```python
from build123d import *

# Parameters (mm, degrees)
SCHIZZO1_W                   = 470
SCHIZZO1_H                   = 100
SCHIZZO1_R                   = 35
ESTRUSIONE_ESTRUSIONE1_DEPTH = 5
FORO_PER_VITE_M8_1_D         = 8.5
RIPETIZIONECIRCOLARE1_COUNT  = 8
SCHIZZO6_R                   = 28
TAGLIO_ESTRUSIONE1_DEPTH     = 3
SMUSSO1_SIZE                 = 0.5
SCHIZZO7_R                   = 2.75
TAGLIO_ESTRUSIONE2_DEPTH     = 424.083916026
RIPETIZIONECIRCOLARE2_COUNT  = 6
RACCORDO1_R                  = 20
RACCORDO2_R                  = 50
TAGLIO_ESTRUSIONE3_START     = -10
TAGLIO_ESTRUSIONE3_DEPTH     = 4
SCHIZZO10_R                  = 2.1
TAGLIO_ESTRUSIONE4_DEPTH     = 424.083916026
SCHIZZO11_R                  = 3.4
TAGLIO_ESTRUSIONE5_DEPTH     = 10
SCHIZZO12_R                  = 2.1
TAGLIO_ESTRUSIONE6_DEPTH     = 424.083916026
TAGLIO_ESTRUSIONE7_DEPTH     = 424.008274151


with BuildPart() as part:
    # Schizzo1 → Estrusione-Estrusione1 (new, symmetric)
    with BuildSketch(Plane(origin=(0, 0, 0), x_dir=(1, 0, 0), z_dir=(0, 1, 0))):
        with Locations((-185, 0)):
            Rectangle(SCHIZZO1_W, SCHIZZO1_H)
        with Locations(Location((-370, 0, 0), (0, 0, 270))):
            Circle(SCHIZZO1_R, mode=Mode.SUBTRACT)
    extrude(amount=ESTRUSIONE_ESTRUSIONE1_DEPTH, both=True)

    # Foro per Vite M8-1 (through all)
    with Locations(Plane(origin=(0, 5, 0), x_dir=(1, 0, 0), z_dir=(0, 1, 0))):
        with Locations((21, 0)):
            foro_per_vite_m8_1 = Hole(FORO_PER_VITE_M8_1_D / 2)

    # RipetizioneCircolare1: Foro per Vite M8-1 ×8 about axis
    ripetizionecircolare1_axis = Axis((0, 0, 0), (0, 1, 0))
    for i in range(1, RIPETIZIONECIRCOLARE1_COUNT):
        add(foro_per_vite_m8_1.rotate(ripetizionecircolare1_axis, i * 360 / RIPETIZIONECIRCOLARE1_COUNT), mode=Mode.SUBTRACT)

    # Schizzo6 → Taglio-Estrusione1 (cut)
    with BuildSketch(Plane.XZ.offset(5)):
        with Locations(Location((0, 0, 0), (0, 0, 270))):
            Circle(SCHIZZO6_R)
    extrude(amount=-TAGLIO_ESTRUSIONE1_DEPTH, mode=Mode.SUBTRACT)

    # Smusso1
    smusso1_edges = [part.edges().sort_by_distance(p)[0] for p in [
        (0, -5, 28),
    ]]
    chamfer(smusso1_edges, length=SMUSSO1_SIZE)

    # Schizzo7 → Taglio-Estrusione2 (cut, through all)
    with BuildSketch(Plane(origin=(0, 5, 0), x_dir=(1, 0, 0), z_dir=(0, 1, 0))):
        with Locations(Location((-370, 41, 0), (0, 0, 270))):
            Circle(SCHIZZO7_R)
    taglio_estrusione2 = extrude(amount=-TAGLIO_ESTRUSIONE2_DEPTH, mode=Mode.SUBTRACT)

    # RipetizioneCircolare2: Taglio-Estrusione2 ×6 about axis
    ripetizionecircolare2_axis = Axis((-370, 0, 0), (0, 1, 0))
    for i in range(1, RIPETIZIONECIRCOLARE2_COUNT):
        add(taglio_estrusione2.rotate(ripetizionecircolare2_axis, i * 360 / RIPETIZIONECIRCOLARE2_COUNT), mode=Mode.SUBTRACT)

    # Raccordo1
    raccordo1_edges = [part.edges().sort_by_distance(p)[0] for p in [
        (50, 0, -50),
        (50, 0, 50),
    ]]
    fillet(raccordo1_edges, radius=RACCORDO1_R)

    # Raccordo2
    raccordo2_edges = [part.edges().sort_by_distance(p)[0] for p in [
        (-420, 0, -50),
        (-420, 0, 50),
    ]]
    fillet(raccordo2_edges, radius=RACCORDO2_R - 0.0001)  # a hair under: the kernel refuses the full size

    # Schizzo9 → Taglio-Estrusione3 (cut)
    with BuildSketch(Plane(origin=(0, 5, 0), x_dir=(1, 0, 0), z_dir=(0, 1, 0)).offset(TAGLIO_ESTRUSIONE3_START)):
        with BuildLine():
            Line((-32, 46.55), (-20, 46.55))
            ThreePointArc((-20, 46.55), (-15.95, 42.5), (-20, 38.45))
            Line((-20, 38.45), (-32, 38.45))
            ThreePointArc((-32, 38.45), (-36.05, 42.5), (-32, 46.55))
        make_face()
        with BuildLine():
            Line((20, 46.55), (32, 46.55))
            ThreePointArc((32, 46.55), (36.05, 42.5), (32, 38.45))
            Line((32, 38.45), (20, 38.45))
            ThreePointArc((20, 38.45), (15.95, 42.5), (20, 46.55))
        make_face()
        with BuildLine():
            Line((-32, -38.45), (-20, -38.45))
            ThreePointArc((-20, -38.45), (-15.95, -42.5), (-20, -46.55))
            Line((-20, -46.55), (-32, -46.55))
            ThreePointArc((-32, -46.55), (-36.05, -42.5), (-32, -38.45))
        make_face()
        with BuildLine():
            Line((20, -38.45), (32, -38.45))
            ThreePointArc((32, -38.45), (36.05, -42.5), (32, -46.55))
            Line((32, -46.55), (20, -46.55))
            ThreePointArc((20, -46.55), (15.95, -42.5), (20, -38.45))
        make_face()
    extrude(amount=TAGLIO_ESTRUSIONE3_DEPTH, mode=Mode.SUBTRACT)

    # Schizzo10 → Taglio-Estrusione4 (cut, through all)
    with BuildSketch(Plane(origin=(0, 5, 0), x_dir=(1, 0, 0), z_dir=(0, 1, 0))):
        with Locations(Location((-150, 0, 0), (0, 0, 270))):
            Circle(SCHIZZO10_R)
    extrude(amount=-TAGLIO_ESTRUSIONE4_DEPTH, mode=Mode.SUBTRACT)

    # Schizzo11 → Taglio-Estrusione5 (cut)
    with BuildSketch(Plane(origin=(0, 5, 0), x_dir=(1, 0, 0), z_dir=(0, 1, 0))):
        with Locations(Location((-280, 43.588989435, 0), (0, 0, 270))):
            Circle(SCHIZZO11_R)
    extrude(amount=-TAGLIO_ESTRUSIONE5_DEPTH, mode=Mode.SUBTRACT)

    # Schizzo12 → Taglio-Estrusione6 (cut, through all)
    with BuildSketch(Plane(origin=(0, 5, 0), x_dir=(1, 0, 0), z_dir=(0, 1, 0))):
        with Locations(Location((-50, -42.5, 0), (0, 0, 270))):
            Circle(SCHIZZO12_R)
        with Locations(Location((-300, -42.5, 0), (0, 0, 270))):
            Circle(SCHIZZO12_R)
        with Locations(Location((-175, -42.5, 0), (0, 0, 270))):
            Circle(SCHIZZO12_R)
    extrude(amount=-TAGLIO_ESTRUSIONE6_DEPTH, mode=Mode.SUBTRACT)

    # Schizzo13 → Taglio-Estrusione7 (cut, through all)
    with BuildSketch(Plane(origin=(0, -1, 0), x_dir=(-1, 0, 0), z_dir=(0, -1, 0))):
        with BuildLine():
            Line((32, -45.25), (20, -45.25))
            ThreePointArc((20, -45.25), (17.25, -42.5), (20, -39.75))
            Line((20, -39.75), (32, -39.75))
            ThreePointArc((32, -39.75), (34.75, -42.5), (32, -45.25))
        make_face()
        with BuildLine():
            Line((-20, -45.25), (-32, -45.25))
            ThreePointArc((-32, -45.25), (-34.75, -42.5), (-32, -39.75))
            Line((-32, -39.75), (-20, -39.75))
            ThreePointArc((-20, -39.75), (-17.25, -42.5), (-20, -45.25))
        make_face()
        with BuildLine():
            Line((-32, 45.25), (-20, 45.25))
            ThreePointArc((-20, 45.25), (-17.25, 42.5), (-20, 39.75))
            Line((-20, 39.75), (-32, 39.75))
            ThreePointArc((-32, 39.75), (-34.75, 42.5), (-32, 45.25))
        make_face()
        with BuildLine():
            Line((20, 45.25), (32, 45.25))
            ThreePointArc((32, 45.25), (34.75, 42.5), (32, 39.75))
            Line((32, 39.75), (20, 39.75))
            ThreePointArc((20, 39.75), (17.25, 42.5), (20, 45.25))
        make_face()
    extrude(amount=-TAGLIO_ESTRUSIONE7_DEPTH, mode=Mode.SUBTRACT)


solid = part.part
```
Can you work these out from the model? Positions are in its coordinate system, mm. A direction names the side the tool comes from. Coordinates: 2 decimals unless noted, no trailing zeros. Answer as CSV lines item,"result".
Item 1: I'm going to push flat-ended pins straight in: P1, Ø4, axis at x = -22.5, z = 41, coming from the -Y side; P2, Ø3.5, axis at x = -370, z = 41, coming from the +Y side; P3, Ø13.5, axis at x = -21, z = 0, coming from the -Y side. Where does each tip first touch, or does it pass through?
Geometry results:
P1,"stops at y = -1"
P2,"passes through"
P3,"stops at y = -2"
Item 2: Please list where these lines run through material, in increasing order: line 1 along X through (y, z) = (-3.5, -39); line 2 along X through (y, z) = (1, 20.5); line 3 along X through (y, z) = (-2.75, 19.5).
Geometry results:
line 1,"x = -401.29 to -371.89, -368.11 to -34.04, -17.96 to 17.96, 34.04 to 47.86"
line 2,"x = -415.6 to -408.26, -402.76 to -398.37, -341.63 to -337.24, -331.74 to -4.22, 4.22 to 50"
line 3,"x = -416.04 to -408.07, -402.95 to -399.06, -340.94 to -337.05, -331.93 to -20.09, 20.09 to 50"
Item 3: On a 3-axis mill with a long thin cutter (end or side, diameter ignored), from which of +Z, -Z, +X, -X, +Y, -Y can I reach the whole of each face in a straight line? I mean faces 1 (the flat face through (26, -1, 39)), 2 (the flat face through (-188, -5, -1)). Say none if no direction works.
Geometry results:
face 1,"-Y"
face 2,"+Z, -Z, +X, -X, -Y"
Item 4: We'd pull the mould along X, two halves only. Please class faces 3 (the cylindrical face through (43.986, -0.07, -44.297)), 4 (the cylindrical face through (-24.132, 1.451, 2.872)), 5 (the cylindrical face through (-404.964, 0.07, 35.742)): +X half, -X half, draft (parallel to the pull), parting line (faces both ways), or undercut.
Geometry results:
face 3,"+X half"
face 4,"undercut"
face 5,"-X half"
Item 5: Imagine slicing it at A-A on y = 3.5. State how many separate pieces and enclosed holes the cut face has, plus the area to 3 significant figures.
Geometry results:
separate pieces,"1"
enclosed holes,"24"
area,"40,900 mm2"
